```python
from build123d import *

# Parameters (mm, degrees)
SKETCH_1_W      = 13
SKETCH_1_H      = 22.18
EXTRUDE_1_DEPTH = 2
SKETCH_2_W      = 13
SKETCH_2_H      = 22.18
EXTRUDE_3_DEPTH = 1


with BuildPart() as part:
    # 草图1 → 凸台-拉伸1 (new body)
    with BuildSketch(Plane.XY):
        with Locations((3.5, -8.09)):
            Rectangle(SKETCH_1_W, SKETCH_1_H)
        Polygon((0, -5), (0, 0), (2, 0), (2, -3), (7, -3), (7, -5), (7, -9), (5, -9), (2, -9), (2, -16.18), (0, -16.18), (0, -9), (0, -7), (5, -7), (5, -5), (2, -5), align=None, mode=Mode.SUBTRACT)
    extrude(amount=-EXTRUDE_1_DEPTH)

    # 草图2 → 凸台-拉伸3 (add)
    with BuildSketch(Plane.XY):
        with Locations((3.5, -8.09)):
            Rectangle(SKETCH_2_W, SKETCH_2_H)
    extrude(amount=EXTRUDE_3_DEPTH)


solid = part.part
```
Verification items for the finished model (mm, model axes). A direction names the side the tool comes from. Round coordinates to 2 decimals unless told otherwise and drop trailing zeros. Order: outer loops, then holes, each group sorted by start corner. A loop starts at its lowest first (then second) coordinate and runs counter-clockwise, first axis right, second up. Notation, with made-up numbers: (61, 25) -> (87, 25) arc R18 ccw to (87, 53) -> close; hole circle Ø1 at (71.25, 45.25). An arc over 180 degrees is marked (long way). Put each result on its own line as item: value. Start each with the question number.
(1) Material ranges on line 1 along Y through (x, z) = (1.25, -0.85); line 2 along Y through (x, z) = (3, -0.8); line 3 along X through (y, z) = (-4.75, -0.9), recorded low to high.
(2) Section check D-D (y = -11.25). Enter the section's corners in (x, z).
(3) Section check B-B (y = -4.5). Enter the section's corners in (x, z).
(4) Section check C-C (z = -1.5). Enter the section's corners in (x, y), then the cut area to 3 significant figures.
(5) Section check A-A (x = 1.25). Enter the section's corners in (y, z), then the cut area to 3 significant figures.
(6) Tool access check on faces 1 (the face through (4, -3, -1)), 2 (the face through (10, -8, -1)). Record the directions out of +Z, -Z, +X, -X, +Y, -Y that give a thin tool (end or side, any length) a straight path to the whole face; none if there is none.
(7) Draft check along X on faces 3 (the face through (3, 3, -1)), 4 (the face through (-3, -8, -1)), 5 (the face through (1, -16.18, -1)). Enter one of: +X half, -X half, draft (parallel to the pull), parting line (faces both ways), or undercut.
Completed:
1. line 1: y = -19.18 to -16.18, -7 to -5, 0 to 3
1. line 2: y = -19.18 to -9, -7 to -5, -3 to 3
1. line 3: x = -3 to 0, 7 to 10
2. outline: (-3, -2) -> (0, -2) -> (0, 0) -> (2, 0) -> (2, -2) -> (10, -2) -> (10, 1) -> (-3, 1) -> close
3. outline: (-3, -2) -> (0, -2) -> (0, 0) -> (7, 0) -> (7, -2) -> (10, -2) -> (10, 1) -> (-3, 1) -> close
4. outline: (-3, -19.18) -> (10, -19.18) -> (10, 3) -> (-3, 3) -> close; hole (0, -16.18) -> (2, -16.18) -> (2, -9) -> (7, -9) -> (7, -3) -> (2, -3) -> (2, 0) -> (0, 0) -> (0, -5) -> (5, -5) -> (5, -7) -> (0, -7) -> close
4. area: 236 mm2
5. outline: (-19.18, -2) -> (-16.18, -2) -> (-16.18, 0) -> (-7, 0) -> (-7, -2) -> (-5, -2) -> (-5, 0) -> (0, 0) -> (0, -2) -> (3, -2) -> (3, 1) -> (-19.18, 1) -> close
5. area: 38.2 mm2
6. face 1: -Z
6. face 2: +Z, -Z, +X, +Y, -Y
7. face 3: draft
7. face 4: -X half
7. face 5: undercut
